from build123d import *

# Parameters (mm, degrees)
F1_DEPTH    = 10
F2_T1_DEPTH = 20
F4_DEPTH    = 20.001
F5_W        = 35
F5_H        = 5
F6_DEPTH    = 10.001
F7_R        = 3
F9_DEPTH    = 10.001
F11_DEPTH   = 4
F12_R       = 5.5
F13_DEPTH   = 2
F14_R       = 4.25
F15_DEPTH   = 112.584302492
F16_R       = 1.395
F17_DEPTH   = 25


# Not quite as in the source:
# - a fillet or chamfer that OpenCascade refuses, or shapes differently, is made with other operations: its cross-section is extruded or revolved along the edge and cut away or added


with BuildPart() as f1:
    # F0 (on Front) → F1 (new body, symmetric)
    with BuildSketch(Plane.XZ):
        with BuildLine():
            Line((30, 51.9615242271), (0, 0))
            Line((0, 0), (130, 0))
            Line((130, 0), (130, 10))
            Line((130, 10), (95, 10))
            ThreePointArc((95, 10), (89.8236190979, 10.6814834742), (85, 12.6794919243))
            Line((85, 12.6794919243), (62.0314784198, 25.9403740415))
            Line((62.0314784198, 25.9403740415), (63.2814784198, 28.105437551))
            Line((63.2814784198, 28.105437551), (45.9609703441, 38.105437551))
            Line((45.9609703441, 38.105437551), (44.7109703441, 35.9403740415))
            Line((44.7109703441, 35.9403740415), (28.0394191624, 45.5656986041))
            Line((28.0394191624, 45.5656986041), (31.2990381057, 51.2115242271))
            Line((31.2990381057, 51.2115242271), (30, 51.9615242271))
        make_face()
    extrude(amount=F1_DEPTH, both=True)

    # F2: fillet of radius 3 on 3 edges, made by hand

    # F2_s2 → F2_t1 (join)
    with BuildSketch(Plane.XZ.offset(-10)):
        with BuildLine():
            ThreePointArc((63.2814784198, 28.105437551), (63.2705212044, 26.0433626604), (64.5932161113, 24.4613540958))
            Line((64.5932161113, 24.4613540958), (62.0314784198, 25.9403740415))
            Line((62.0314784198, 25.9403740415), (63.2814784198, 28.105437551))
        make_face()
        with BuildLine():
            ThreePointArc((42.1492326526, 37.4193939873), (44.180639712, 37.0649108788), (45.9609703441, 38.105437551))
            Line((45.9609703441, 38.105437551), (44.7109703441, 35.9403740415))
            Line((44.7109703441, 35.9403740415), (42.1492326526, 37.4193939873))
        make_face()
        with BuildLine():
            ThreePointArc((29.5394191624, 48.1637748154), (29.2397178949, 45.8873176801), (30.6374953738, 44.0656986041))
            Line((30.6374953738, 44.0656986041), (28.0394191624, 45.5656986041))
            Line((28.0394191624, 45.5656986041), (29.5394191624, 48.1637748154))
        make_face()
    extrude(amount=F2_T1_DEPTH)

    # F3 (on face) → F4 (cut, through all)
    with BuildSketch(Plane.XZ.offset(10)):
        with BuildLine():
            ThreePointArc((82.7031939779, 1.5), (87.5328231093, 5.2059047745), (85.2031939779, 10.8301270189))
            Line((85.2031939779, 10.8301270189), (31.6195461814, 41.7666604984))
            ThreePointArc((31.6195461814, 41.7666604984), (27.8254509559, 42.2661626109), (24.7894191624, 39.9365334795))
            Line((24.7894191624, 39.9365334795), (11.2990381057, 16.5705080757))
            ThreePointArc((11.2990381057, 16.5705080757), (10.7995359932, 12.7764128502), (13.1291651246, 9.7403810568))
            Line((13.1291651246, 9.7403810568), (27.4019237886, 1.5))
            Line((27.4019237886, 1.5), (82.7031939779, 1.5))
        make_face()
    extrude(amount=-F4_DEPTH, mode=Mode.SUBTRACT)

    # F5 (on face) → F6 (cut, through all)
    with BuildSketch(Plane.XY.offset(10)):
        with Locations((112.5, 7.5)):
            Rectangle(F5_W, F5_H)
        with Locations((112.5, -7.5)):
            Rectangle(F5_W, F5_H)
    extrude(amount=-F6_DEPTH, mode=Mode.SUBTRACT)

    # F7
    f7_edges = [f1.edges().sort_by_distance(p)[0] for p in [
        (95, -5, 5),
        (95, 5, 5),
    ]]
    fillet(f7_edges, radius=F7_R)

    # F8 (on face) → F9 (cut, through all)
    with BuildSketch(Plane.XY.offset(10)):
        with BuildLine():
            Line((130, -3), (130, 3))
            Line((130, 3), (113, 3))
            ThreePointArc((113, 3), (110, 0), (113, -3))
            Line((113, -3), (130, -3))
        make_face()
    extrude(amount=-F9_DEPTH, mode=Mode.SUBTRACT)

    # F10 (on face) → F11 (cut)
    with BuildSketch(Plane(origin=(27.9903810568, 0, 48.4807621135), x_dir=(0.8660254038, 0, -0.5), z_dir=(0.5, 0, 0.8660254038))):
        with BuildLine():
            Line((35, 4), (28, 4))
            ThreePointArc((28, 4), (24, 0), (28, -4))
            Line((28, -4), (35, -4))
            ThreePointArc((35, -4), (39, 0), (35, 4))
        make_face()
    extrude(amount=-F11_DEPTH, mode=Mode.SUBTRACT)

    # F12 (on face) → F13 (cut)
    with BuildSketch(Plane(origin=(0, 0, 0), x_dir=(0, -1, 0), z_dir=(-0.8660254038, 0, 0.5))):
        with Locations((0, 7.5)):
            Circle(F12_R)
    extrude(amount=-F13_DEPTH, mode=Mode.SUBTRACT)

    # F14 (on face) → F15 (cut, through all)
    with BuildSketch(Plane(origin=(0, 0, 0), x_dir=(0, -1, 0), z_dir=(-0.8660254038, 0, 0.5))):
        with Locations((0, 7.5)):
            Circle(F14_R)
    extrude(amount=-F15_DEPTH, mode=Mode.SUBTRACT)

    # F16 (on face) → F17 (cut)
    with BuildSketch(Plane(origin=(0, 0, 0), x_dir=(0, -1, 0), z_dir=(-0.8660254038, 0, 0.5))):
        with Locations((-5, 25)):
            Circle(F16_R)
        with Locations((-5, 32)):
            Circle(F16_R)
        with Locations((-5, 39)):
            Circle(F16_R)
        with Locations((5, 39)):
            Circle(F16_R)
        with Locations((5, 32)):
            Circle(F16_R)
        with Locations((5, 25)):
            Circle(F16_R)
    extrude(amount=-F17_DEPTH, mode=Mode.SUBTRACT)


solid = f1.part
Geometry check sheet. Reference: the model listing, model coordinates, mm. A direction names the side the tool comes from. Round coordinates to 2 decimals unless told otherwise and drop trailing zeros. Loops run counter-clockwise (first coordinate to the right, second up) from the corner with the lowest first, then second, coordinate; pieces in that order, holes last.
Item 1: Thickness scan on line 1 (Z direction, x = 121.5, y = 4.75); line 2 (X direction, y = -1.5, z = 19); line 3 (Y direction, x = 98, z = 3). Record the ranges inside material, lowest first.
Item 2: Cross-section at C-C on x = 106.5. Record the boundary of the cut face in (y, z).
Item 3: Mould release check, pull along Y, two halves, no side actions. Record for faces 1 (the flat face through (114, 5, 5)), 2 (the flat face through (15.21, -0.14, 26.344)), 3 (the cylindrical face through (60.779, -0.088, 27.273)), 4 (the flat face through (54, -4, 31)): pulls with the +Y half, pulls with the -Y half, needs draft (parallel to the pull), parting line crosses it, or undercut.
Item 4: Access from +Z, -Z, +X, -X, +Y, -Y to the whole of each face (thin tool, end or side, straight path). Record for faces 5 (the cylindrical face through (44.15, 0.14, 37.06)), 6 (the flat face through (30.41, -0.14, 49.67)), 7 (the flat face through (58.79, -4.58, 26.08)).
Item 5: Cross-section at B-B on x = 55. Record the boundary of the cut face in (y, z).
Item 6: Gauge pin test, flat ends, axial feed: pin 1 (5 mm diameter, centred on x = 36, y = -2.5, fed in from -Z); pin 2 (5 mm diameter, centred on x = 122, z = 7, fed in from -Y); pin 3 (2 mm diameter, centred on y = -9, z = 6, fed in from +X); pin 4 (10 mm diameter, centred on y = 2.5, z = 41, fed in from +X). Record the tip position at first contact, or that the pin passes through.
Answer sheet:
1. line 1: z = 0 to 10
1. line 2: x = 10.97 to 12.7, 71.05 to 74.05
1. line 3: y = -5 to 5
2. outline: (-5, 0) - (5, 0) - (5, 10) - (-5, 10) - close
3. face 1: pulls with the +Y half
3. face 2: needs draft
3. face 3: undercut
3. face 4: undercut
4. face 5: +Z, +Y, -Y
4. face 6: +X, +Y, -Y
4. face 7: +Y, -Y
5. outline: (-10, 0) - (10, 0) - (10, 1.5) - (-10, 1.5) - close; (-10, 28.27) - (-4, 28.27) - (-4, 32.89) - (-10, 32.89) - close; (4, 28.27) - (10, 28.27) - (10, 32.89) - (4, 32.89) - close
6. pin 1: stops at z = 0
6. pin 2: stops at y = -5
6. pin 3: stops at x = 95
6. pin 4: stops at x = 49.61
